Input: dimensioned drawing with shaded views. Units: mm. Origin: part minimum x, y, z. Round coordinates to 2 decimals unless told otherwise and drop trailing zeros. Loops run counter-clockwise (first coordinate to the right, second up) from the corner with the lowest first, then second, coordinate; pieces in that order, holes last. Notation, with made-up numbers: (44, 69) -> (71, 69) arc R19 ccw to (71, 98) -> close; hole circle Ø7 at (7, -23). An arc over 180 degrees is marked (long way). Answer as a JSON object with one key per item and string values.
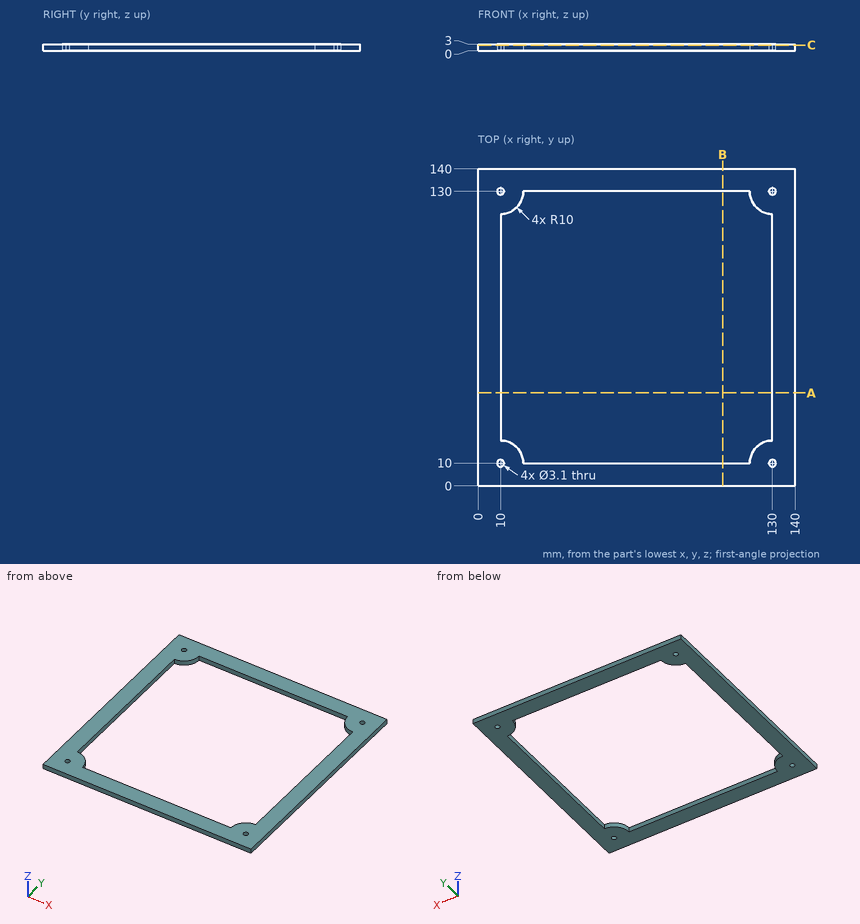
1) Section A-A, the plane y = 41. Output: boundary loops of the cut face in (x, z).
Output:
{"outline": "(0, 0) -> (10, 0) -> (10, 3) -> (0, 3) -> close; (130, 0) -> (140, 0) -> (140, 3) -> (130, 3) -> close"}
2) Contact query for flat-ended pins moving along their axis: P1, Ø1, axis at x = 89, z = 1, coming from the -Y side; P2, Ø1.9, axis at x = 130, y = 10, coming from the -Z side. Output: stop coordinate, or through.
Output:
{"P1": "stops at y = 0", "P2": "passes through"}
3) Section C-C, the plane z = 2.55. Output: boundary loops of the cut face in (x, y), plus the area to 3 significant figures.
Output:
{"outline": "(0, 0) -> (140, 0) -> (140, 140) -> (0, 140) -> close; hole circle Ø3.1 at (10, 10); hole circle Ø3.1 at (10, 130); hole (10, 20) arc R10 cw to (20, 10) -> (120, 10) arc R10 cw to (130, 20) -> (130, 120) arc R10 cw to (120, 130) -> (20, 130) arc R10 cw to (10, 120) -> close; hole circle Ø3.1 at (130, 10); hole circle Ø3.1 at (130, 130)", "area": "5,480 mm^2"}
4) Ray query, probe 1 along X at (y, z) = (31, 2.2); probe 2 along X at (y, z) = (9, 1.3). Return the intervals inside material, ascending.
Output:
{"probe 1": "x = 0 to 10, 130 to 140", "probe 2": "x = 0 to 8.82, 11.18 to 128.82, 131.18 to 140"}
